```python
from build123d import *

# Parameters (mm, degrees)
SKETCH1_R               = 2.65
BOSS_EXTRUDE1_DEPTH     = 9
SKETCH2_W               = 5
SKETCH2_H               = 70
BOSS_EXTRUDE2_DEPTH     = 10
SKETCH3_R               = 1.65
CUT_EXTRUDE1_DEPTH      = 10
SKETCH4_R               = 3.75
CUT_EXTRUDE2_DEPTH      = 3
CUT_EXTRUDE3_DEPTH      = 3
CHAMFER1_SIZE           = 4
CUT_EXTRUDE4_DEPTH      = 5
CUT_EXTRUDE4_DEPTH_BACK = 4
SKETCH6_R               = 5


with BuildPart() as part:
    # Sketch1 → Boss-Extrude1 (new body)
    with BuildSketch(Plane(origin=(0, 0, 0), x_dir=(1, 0, 0), z_dir=(0, 1, 0))):
        with BuildLine():
            Line((57, 70), (57, 49.8))
            Line((57, 49.8), (42, 49.8))
            Line((42, 49.8), (42, 0))
            Line((42, 0), (37, 0))
            ThreePointArc((37, 0), (21, 16), (5, 0))
            Line((5, 0), (0, 0))
            Line((0, 0), (0, 49.8))
            Line((0, 49.8), (-15, 49.8))
            Line((-15, 49.8), (-15, 70))
            Line((-15, 70), (0, 70))
            Line((0, 70), (57, 70))
        make_face()
        with Locations(Location((-7.5, 59.9, 0), (0, 0, 270))):
            Circle(SKETCH1_R, mode=Mode.SUBTRACT)
        with Locations(Location((49.5, 59.9, 0), (0, 0, 270))):
            Circle(SKETCH1_R, mode=Mode.SUBTRACT)
    extrude(amount=BOSS_EXTRUDE1_DEPTH)

    # Sketch2 → Boss-Extrude2 (add)
    with BuildSketch(Plane(origin=(0, 9, 0), x_dir=(1, 0, 0), z_dir=(0, 1, 0))):
        with Locations((2.5, 35)):
            Rectangle(SKETCH2_W, SKETCH2_H)
        with Locations((39.5, 35)):
            Rectangle(SKETCH2_W, SKETCH2_H)
    extrude(amount=BOSS_EXTRUDE2_DEPTH)

    # Sketch3 → Cut-Extrude1 (cut)
    with BuildSketch(Plane.XZ):
        with Locations(Location((13, -24, 0), (0, 0, 270))):
            Circle(SKETCH3_R)
        with Locations(Location((29, -24, 0), (0, 0, 270))):
            Circle(SKETCH3_R)
    extrude(amount=-CUT_EXTRUDE1_DEPTH, mode=Mode.SUBTRACT)

    # Sketch4 → Cut-Extrude2 (cut)
    with BuildSketch(Plane(origin=(0, 9, 0), x_dir=(1, 0, 0), z_dir=(0, 1, 0))):
        with Locations(Location((13, 24, 0), (0, 0, 270))):
            Circle(SKETCH4_R)
        with Locations(Location((29, 24, 0), (0, 0, 270))):
            Circle(SKETCH4_R)
    extrude(amount=-CUT_EXTRUDE2_DEPTH, mode=Mode.SUBTRACT)

    # Sketch5 → Cut-Extrude3 (cut)
    with BuildSketch(Plane(origin=(0, 9, 0), x_dir=(1, 0, 0), z_dir=(0, 1, 0))):
        with BuildLine():
            Line((16.5, 19), (25.5, 19))
            ThreePointArc((25.5, 19), (28.5, 16), (25.5, 13))
            Line((25.5, 13), (16.5, 13))
            ThreePointArc((16.5, 13), (13.5, 16), (16.5, 19))
        make_face()
    extrude(amount=-CUT_EXTRUDE3_DEPTH, mode=Mode.SUBTRACT)

    # Chamfer1
    chamfer1_edges = [part.edges().sort_by_distance(p)[0] for p in [
        (42, 4.5, -49.8),
        (0, 4.5, -49.8),
        (0, 9, -59.9),
        (42, 9, -59.9),
    ]]
    chamfer(chamfer1_edges, length=CHAMFER1_SIZE)

    # Sketch6 → Cut-Extrude4 (cut, two sides: drawn at the far end of the back side and taken through both)
    with BuildSketch(Plane(origin=(0, 9, 0), x_dir=(1, 0, 0), z_dir=(0, 1, 0)).offset(-CUT_EXTRUDE4_DEPTH_BACK)):
        with Locations(Location((-7.5, 59.9, 0), (0, 0, 45.572995999))):
            Circle(SKETCH6_R)
        with Locations(Location((49.5, 59.9, 0), (0, 0, 134.427004001))):
            Circle(SKETCH6_R)
    extrude(amount=CUT_EXTRUDE4_DEPTH + CUT_EXTRUDE4_DEPTH_BACK, mode=Mode.SUBTRACT)


solid = part.part
```
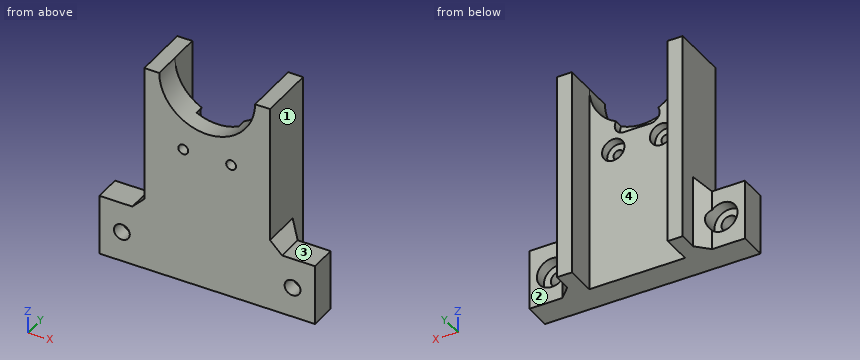
Part model, mm, in its own coordinate system. Face numbers are marked on the shaded views. A direction names the side the tool comes from. Give positions to 0.01 mm unless a question says otherwise; leave off trailing zeros. Order: outer loops, then holes, each group sorted by start corner. A loop starts at its lowest first (then second) coordinate and runs counter-clockwise, first axis right, second up. Notation, with made-up numbers: M 10,-35 L 65,-35 A25 cw 65,-4 Z; hole C -38,57 d11. An arc over 180 degrees is marked long. Use a Markdown table: item, result. Add a question column.
(1) Saw through at A-A, the plane y = 16.25. Give the cut face in (x, z).
(2) Saw through at B-B, the plane z = -24. Give the cut face in (x, y), and give its area (3 significant figures).
(3) Saw through at C-C, the plane x = 49.5. Give the cut face in (y, z).
(4) Drop flat-ended pins along their axis: P1, Ø2.5, axis at x = 23, y = 7, coming from the +Z side; P2, Ø3.5, axis at x = -11, z = -62.5, coming from the +Y side; P3, Ø10, axis at x = 49.5, y = 13, coming from the +Z side. Give the stop position or say it passes through.
(5) 3-axis set-ups, long thin cutter, end or side, ignore diameter. For the marked faces 1, 2, 3 and 4: which of +Z, -Z, +X, -X, +Y, -Y reach the whole face in a straight line?
(6) Probe line 1 along X through (y, z) = (6.7, -24); line 2 along X through (y, z) = (4.7, -24); line 3 along Z through (x, y) = (49.5, 3.3). List the from-to ranges inside material, lowest first. Write a range as [from, to].
(7) Saw through at D-D, the plane y = 2. Give the cut face in (x, z).
Answer key:
| question | item | result |
|---|---|---|
| 1 | outline | M 0,-70 L 5,-70 L 5,0 L 0,0 Z; M 37,-70 L 42,-70 L 42,0 L 37,0 Z |
| 2 | outline | M 0,0 L 11.35,0 L 11.35,6 L 9.25,6 L 9.25,9 L 5,9 L 5,19 L 0,19 Z; M 14.65,0 L 27.35,0 L 27.35,6 L 25.25,6 L 25.25,9 L 16.75,9 L 16.75,6 L 14.65,6 Z; M 30.65,0 L 42,0 L 42,19 L 37,19 L 37,9 L 32.75,9 L 32.75,6 L 30.65,6 Z |
| 2 | area | 393 mm^2 |
| 3 | outline | M 0,-70 L 9,-70 L 9,-64.9 L 5,-64.9 L 5,-62.55 L 0,-62.55 Z; M 0,-57.25 L 5,-57.25 L 5,-54.9 L 9,-54.9 L 9,-49.8 L 0,-49.8 Z |
| 4 | P1 | z = -15.76 |
| 4 | P2 | y = 9 |
| 4 | P3 | z = -49.8 |
| 5 | face 1 | +Z, +X, +Y |
| 5 | face 2 | +Z, -Z, +X, +Y |
| 5 | face 3 | +Z, +X, +Y, -Y |
| 5 | face 4 | +Z, -Z, +Y |
| 6 | line 1 | [0, 9.25], [16.75, 25.25], [32.75, 42] |
| 6 | line 2 | [0, 11.35], [14.65, 27.35], [30.65, 42] |
| 6 | line 3 | [-70, -62.55], [-57.25, -49.8] |
| 7 | outline | M -15,-70 L 57,-70 L 57,-49.8 L 46,-49.8 L 42,-45.8 L 42,0 L 37,0 A16 cw 5,0 L 0,0 L 0,-45.8 L -4,-49.8 L -15,-49.8 Z; hole C -7.5,-59.9 d5.3; hole C 13,-24 d3.3; hole C 29,-24 d3.3; hole C 49.5,-59.9 d5.3 |
